```python
from build123d import *

# Parameters (mm, degrees)
SKETCH005_R  = 2.5
PAD003_DEPTH = 49
SKETCH002_R  = 11
PAD001_DEPTH = 10
SKETCH003_R  = 1.5
POCKET_DEPTH = 4.5
PAD_DEPTH    = 15
PAD002_DEPTH = 10


with BuildPart() as shaft:
    # Sketch005 → Pad003 (new body)
    with BuildSketch(Plane.XZ):
        Circle(SKETCH005_R)
    extrude(amount=PAD003_DEPTH)


with BuildPart() as front_holes:
    # Sketch002 → Pad001 (new body)
    with BuildSketch(Plane.XZ.offset(15)):
        Polygon((-21.05, -16.05), (-21.05, 16.05), (-16.05, 21.05), (16.05, 21.05), (21.05, 16.05), (21.05, -16.05), (16.05, -21.05), (-16.05, -21.05), align=None)
        Circle(SKETCH002_R, mode=Mode.SUBTRACT)
    extrude(amount=PAD001_DEPTH)

    # Sketch003 → Pocket (cut)
    with BuildSketch(Plane.XZ.offset(25)):
        with Locations((-15.5, 15.5)):
            Circle(SKETCH003_R)
        with Locations((15.5, 15.5)):
            Circle(SKETCH003_R)
        with Locations((-15.5, -15.5)):
            Circle(SKETCH003_R)
        with Locations((15.5, -15.5)):
            Circle(SKETCH003_R)
    extrude(amount=-POCKET_DEPTH, mode=Mode.SUBTRACT)


with BuildPart() as center:
    # Sketch001 → Revolution (revolve)
    with BuildSketch(Plane.YZ):
        Polygon((-24, 12), (0, 12), (0, 0), (-22, 0), (-22, 3.5), (-27, 3.5), (-27, 11), (-24, 11), align=None)
    revolve(axis=Axis((0, 0, 0), (0, 1, 0)))


with BuildPart() as front_middle_center:
    # Sketch → Pad (new body, symmetric)
    with BuildSketch(Plane.XZ):
        Polygon((-21, 13), (-21, -13), (-13, -21), (13, -21), (21, -13), (21, 13), (13, 21), (-13, 21), align=None)
    extrude(amount=PAD_DEPTH, both=True)

    # Fusion: union center
    add(center.part)

    # Fusion001: union front-holes
    add(front_holes.part)


with BuildPart() as nema17:
    # Sketch004 → Pad002 (new body)
    with BuildSketch(Plane(origin=(0, 15, 0), x_dir=(-1, 0, 0), z_dir=(0, 1, 0))):
        Polygon((-21.05, -16.05), (-21.05, 16.05), (-16.05, 21.05), (16.05, 21.05), (21.05, 16.05), (21.05, -16.05), (16.05, -21.05), (-16.05, -21.05), align=None)
    extrude(amount=PAD002_DEPTH)

    # Fusion002: union front-middle-center
    add(front_middle_center.part)

    # Fusion003: union shaft
    add(shaft.part)


solid = nema17.part
```
Design review of the part built by this model. Coordinates are the model's own, in mm. A direction names the side the tool comes from. Coordinates: 2 decimals unless noted, no trailing zeros. Order: outer loops, then holes, each group sorted by start corner. A loop starts at its lowest first (then second) coordinate and runs counter-clockwise, first axis right, second up.
1) Take a section at D-D, the plane x = -4.5. Give the boundary of the cut face in (y, z), and give its area (3 significant figures).
2) Take a section at B-B, the plane y = 18.5. Give the boundary of the cut face in (x, z).
3) Wall thickness on line 1 along X through (y, z) = (-25.1, 0); line 2 along Z through (x, y) = (15.5, -21.65); line 3 along Z through (x, y) = (-15, -21): over which ranges is each line inside the solid? List them lowest first.
4) Mouldability with a two-part tool opening along X and no side actions: class faces 1 (the flat face through (0, 0, 21)), 2 (the flat face through (-21.05, -20, 0)), 3 (the cylindrical face through (-17, -22.78, 15.57)) as +X half, -X half, draft (parallel to the pull), parting line (faces both ways), or undercut.
5) For faces 4 (the flat face through (15, -20.5, -15)), 5 (the flat face through (17, 0, -17)), 6 (the flat face through (-17, 0, 17)), 7 (the flat face through (17.3, -15, -17.1)), list the 3-axis set-ups (+Z, -Z, +X, -X, +Y, -Y) from which the entire face can be reached by the end or side of a thin tool; tool diameter is ignored.
6) Clearance check with flat-ended pins moving along their axes: pin 1 (1.5 mm diameter, centred on x = 15.5, z = -15, fed in from -Y); pin 2 (2 mm diameter, centred on x = 12.5, z = 2.5, fed in from -Y); pin 3 (1.5 mm diameter, centred on x = 8, y = 4, fed in from +Z); pin 4 (1.5 mm diameter, centred on x = -5, y = -38, fed in from -Z). State where each tip first meets the part, or that it passes through.
7) Take a section at A-A, the plane y = -23. Give the boundary of the cut face in (x, z).
8) Take a section at C-C, the plane z = 0. Give the boundary of the cut face in (x, y), and give its area (3 significant figures).
Returned:
1. outline: (-27, -10.04) - (-25, -10.04) - (-25, -21.05) - (-15, -21.05) - (-15, -21) - (15, -21) - (15, -21.05) - (25, -21.05) - (25, 21.05) - (15, 21.05) - (15, 21) - (-15, 21) - (-15, 21.05) - (-25, 21.05) - (-25, 10.04) - (-27, 10.04) - close
1. area: 2,140 mm2
2. outline: (-21.05, -16.05) - (-16.05, -21.05) - (16.05, -21.05) - (21.05, -16.05) - (21.05, 16.05) - (16.05, 21.05) - (-16.05, 21.05) - (-21.05, 16.05) - close
3. line 1: x = -11 to -3.5, -2.5 to 2.5, 3.5 to 11
3. line 2: z = -21.05 to -17, -14 to 14, 17 to 21.05
3. line 3: z = -21.05 to -16.91, -14.09 to 14.09, 16.91 to 21.05
4. face 1: draft
4. face 2: -X half
4. face 3: undercut
5. face 4: -Y
5. face 5: -Z, +X
5. face 6: +Z, -X
5. face 7: none
6. pin 1: stops at y = -20.5
6. pin 2: stops at y = -25
6. pin 3: stops at z = 21
6. pin 4: passes through
7. outline: (-21.05, -16.05) - (-16.05, -21.05) - (16.05, -21.05) - (21.05, -16.05) - (21.05, 16.05) - (16.05, 21.05) - (-16.05, 21.05) - (-21.05, 16.05) - close; circle Ø5 at (0, 0); hole circle Ø3 at (-15.5, -15.5); hole circle Ø3 at (-15.5, 15.5); hole circle Ø7 at (0, 0); hole circle Ø3 at (15.5, -15.5); hole circle Ø3 at (15.5, 15.5)
8. outline: (-21.05, -25) - (-11, -25) - (-11, -27) - (-3.5, -27) - (-3.5, -22) - (-2.5, -22) - (-2.5, -49) - (2.5, -49) - (2.5, -22) - (3.5, -22) - (3.5, -27) - (11, -27) - (11, -25) - (21.05, -25) - (21.05, -15) - (21, -15) - (21, 15) - (21.05, 15) - (21.05, 25) - (-21.05, 25) - (-21.05, 15) - (-21, 15) - (-21, -15) - (-21.05, -15) - close
8. area: 2,250 mm2
